from build123d import *

# Parameters (mm, degrees)
SKETCH1_W                       = 120
SKETCH1_H                       = 120
SKETCH1_W_2                     = 100
SKETCH1_H_2                     = 100
BOSS_EXTRUDE1_DEPTH             = 100
SKETCH2_W                       = 120
SKETCH2_H                       = 40
SKETCH2_H_2                     = 120
SKETCH2_W_2                     = 100
SKETCH2_H_3                     = 100
BOSS_EXTRUDE2_DEPTH             = 15
F_5_0MM_DOWEL_HOLE2_D           = 5
F_5_0MM_DOWEL_HOLE2_CSINK_D     = 5.05
F_5_0MM_DOWEL_HOLE2_CSINK_ANGLE = 90
F_5_0MM_DOWEL_HOLE1_D           = 5
F_5_0MM_DOWEL_HOLE1_CSINK_D     = 5.05
F_5_0MM_DOWEL_HOLE1_CSINK_ANGLE = 90
FILLET1_R                       = 15
FILLET2_R                       = 10


with BuildPart() as part:
    # Sketch1 → Boss-Extrude1 (new body)
    with BuildSketch(Plane(origin=(0, 0, 0), x_dir=(0, 1, 0), z_dir=(0, 0, 1))):
        Rectangle(SKETCH1_W, SKETCH1_H)
        Rectangle(SKETCH1_W_2, SKETCH1_H_2, mode=Mode.SUBTRACT)
    extrude(amount=BOSS_EXTRUDE1_DEPTH)

    # Sketch2 → Boss-Extrude2 (add)
    # profile 1 of 4: a face of its own
    with BuildSketch(Plane(origin=(0, 0, 0), x_dir=(1, 0, 0), z_dir=(0, 0, -1))):
        with Locations((0, 80)):
            Rectangle(SKETCH2_W, SKETCH2_H)
    # profile 2 of 4: a face of its own
    with BuildSketch(Plane(origin=(0, 0, 0), x_dir=(1, 0, 0), z_dir=(0, 0, -1))):
        with Locations((0, -80)):
            Rectangle(SKETCH2_W, SKETCH2_H)
    # profile 3 of 4: a face of its own
    with BuildSketch(Plane(origin=(0, 0, 0), x_dir=(1, 0, 0), z_dir=(0, 0, -1))):
        Rectangle(SKETCH2_W, SKETCH2_H_2)
        Rectangle(SKETCH2_W_2, SKETCH2_H_3, mode=Mode.SUBTRACT)
    # profile 4 of 4: a face of its own
    with BuildSketch(Plane(origin=(0, 0, 0), x_dir=(1, 0, 0), z_dir=(0, 0, -1))):
        Rectangle(SKETCH2_W_2, SKETCH2_H_3)
    extrude(amount=BOSS_EXTRUDE2_DEPTH)

    # Ø5.0mm Dowel Hole2 (through all)
    with Locations(Plane(origin=(0, 0, -15), x_dir=(1, 0, 0), z_dir=(0, 0, -1))):
        with Locations((37.5, -80), (-37.5, 80), (37.5, 80), (-37.5, -80)):
            CounterSinkHole(F_5_0MM_DOWEL_HOLE2_D / 2, F_5_0MM_DOWEL_HOLE2_CSINK_D / 2, counter_sink_angle=F_5_0MM_DOWEL_HOLE2_CSINK_ANGLE)

    # Ø5.0mm Dowel Hole1 (through all)
    with Locations(Plane(origin=(0, 60, 0), x_dir=(-1, 0, 0), z_dir=(0, 1, 0))):
        with Locations((0, 25)):
            CounterSinkHole(F_5_0MM_DOWEL_HOLE1_D / 2, F_5_0MM_DOWEL_HOLE1_CSINK_D / 2, counter_sink_angle=F_5_0MM_DOWEL_HOLE1_CSINK_ANGLE)

    # Fillet1
    fillet1_edges = [part.edges().sort_by_distance(p)[0] for p in [
        (60, -100, -7.5),
        (-60, -100, -7.5),
        (-60, 100, -7.5),
        (60, 100, -7.5),
    ]]
    fillet(fillet1_edges, radius=FILLET1_R)

    # Fillet2
    fillet2_edges = [part.edges().sort_by_distance(p)[0] for p in [
        (0, 60, 0),
        (0, -60, 0),
    ]]
    fillet(fillet2_edges, radius=FILLET2_R)


solid = part.part
Work out the finished part from the listing and answer in its coordinate system (mm). A direction names the side the tool comes from. Give positions to 0.01 mm unless a question says otherwise; leave off trailing zeros. Order: outer loops, then holes, each group sorted by start corner. A loop starts at its lowest first (then second) coordinate and runs counter-clockwise, first axis right, second up. Notation, with made-up numbers: (-13, -20) -> (29, -20) arc R19 ccw to (29, 15) -> close; hole circle Ø3 at (47.5, -7). An arc over 180 degrees is marked (long way). Answer as a JSON object with one key per item and string values. Group by question number.
1. Section B-B on x = 37.5 is taken. Determine the outline of the cut face in (y, z) (3 decimals).
2. Section C-C on z = 25 is taken. Determine the outline of the cut face in (x, y) (3 decimals), plus the area to 3 significant figures.
3. Consider line 1 along Y through (x, z) = (37.5, -4.75); line 2 along Y through (x, z) = (-37, -11); line 3 along X through (y, z) = (-80, -6). Determine where each line is inside the solid, lowest interval first. Write a range as [from, to].
4. Section D-D on y = 22 is taken. Determine the outline of the cut face in (x, z).
5. The mould has two halves that part along X. Classify faces 1 (the cylindrical face through (-39.81, 80.96, -7.38)), 2 (the cylindrical face through (-0.33, 54.92, 27.48)), 3 (the cylindrical face through (-55.72, 95.49, -7.6)), 4 (the flat face through (-1, 85, 0)): released by +X, released by -X, zero draft, split by the parting line, or undercut.
6. A tool of negligible diameter and unlimited length cuts with its end or side. For faces 5 (the flat face through (50, -1, 49)), 6 (the flat face through (-1, -1, -15)), 7 (the flat face through (1, 60, 54)), from which of +Z, -Z, +X, -X, +Y, -Y can it reach the whole face along a straight path? Write none if from no direction.
7. Section A-A on y = 80 is taken. Determine the outline of the cut face in (x, z) (3 decimals).
8. Flat-ended cylindrical pins translate along their axes: pin 1 Ø6 at (x, y) = (37.5, -80) entering from -Z; pin 2 Ø3 at (x, y) = (13, 67) entering from +Z; pin 3 Ø5 at (x, z) = (41, 50) entering from -Y; pin 4 Ø15 at (x, y) = (-16, -84.5) entering from +Z. Find the tip coordinate at first contact, or state that the pin passes through.
Result sheet:
{
 "1": {"outline": "(-100, -15) -> (-82.525, -15) -> (-82.5, -14.975) -> (-82.5, 0) -> (-100, 0) -> close; (-77.5, -14.975) -> (-77.475, -15) -> (77.475, -15) -> (77.5, -14.975) -> (77.5, 0) -> (70, 0) arc R10 cw to (60, 10) -> (60, 100) -> (50, 100) -> (50, 0) -> (-50, 0) -> (-50, 100) -> (-60, 100) -> (-60, 10) arc R10 cw to (-70, 0) -> (-77.5, 0) -> close; (82.5, -14.975) -> (82.525, -15) -> (100, -15) -> (100, 0) -> (82.5, 0) -> close"},
 "2": {"outline": "(-60, -60) -> (-2.5, -60) -> (-2.5, -50) -> (-50, -50) -> (-50, 50) -> (-2.5, 50) -> (-2.5, 59.975) -> (-2.525, 60) -> (-60, 60) -> close; (2.5, -60) -> (60, -60) -> (60, 60) -> (2.525, 60) -> (2.5, 59.975) -> (2.5, 50) -> (50, 50) -> (50, -50) -> (2.5, -50) -> close", "area": "4,300 mm^2"},
 "3": {"line 1": "y = [-100, -82.5], [-77.5, 77.5], [82.5, 100]", "line 2": "y = [-100, -82.45], [-77.55, 77.55], [82.45, 100]", "line 3": "x = [-60, -40], [-35, 35], [40, 60]"},
 "4": {"outline": "(-60, -15) -> (60, -15) -> (60, 100) -> (50, 100) -> (50, 0) -> (-50, 0) -> (-50, 100) -> (-60, 100) -> close"},
 "5": {"face 1": "undercut", "face 2": "undercut", "face 3": "released by -X", "face 4": "zero draft"},
 "6": {"face 5": "+Z", "face 6": "-Z, +X, -X, +Y, -Y", "face 7": "+Z, +X, -X, +Y"},
 "7": {"outline": "(-60, -15) -> (-40.025, -15) -> (-40, -14.975) -> (-40, 0) -> (-60, 0) -> close; (-35, -14.975) -> (-34.975, -15) -> (34.975, -15) -> (35, -14.975) -> (35, 0) -> (-35, 0) -> close; (40, -14.975) -> (40.025, -15) -> (60, -15) -> (60, 0) -> (40, 0) -> close"},
 "8": {"pin 1": "stops at z = -15", "pin 2": "stops at z = 1.07", "pin 3": "stops at y = -60", "pin 4": "stops at z = 0"}
}
